from build123d import *

# Parameters (mm, degrees)
SKETCH_1_R          = 23
SKETCH_1_R_2        = 18
EXTRUDE_1_DEPTH     = 28
EXTRUDE_3_DEPTH     = 60
SKETCH_2_5_R        = 54
SKETCH_2_5_R_2      = 34
EXTRUDE_4_DEPTH     = 80
CUT_EXTRUDE_1_DEPTH = 30
SKETCH_6_W          = 108
SKETCH_6_H          = 28
EXTRUDE_5_DEPTH     = 60
EXTRUDE_6_DEPTH     = 15


with BuildPart() as part:
    # Sketch 1 → Extrude 1 (new body)
    with BuildSketch(Plane(origin=(0, 0, 0), x_dir=(1, 0, 0), z_dir=(0, 1, 0))):
        with BuildLine():
            Line((0, 40), (180, 40))
            ThreePointArc((180, 40), (220, 0), (180, -40))
            Line((180, -40), (0, -40))
            ThreePointArc((0, -40), (-40, 0), (0, 40))
        make_face()
        with Locations(Location((180, 0, 0), (0, 0, 270))):
            Circle(SKETCH_1_R, mode=Mode.SUBTRACT)
        with Locations(Location((0, 0, 0), (0, 0, 270))):
            Circle(SKETCH_1_R_2, mode=Mode.SUBTRACT)
    extrude(amount=EXTRUDE_1_DEPTH)



with BuildPart() as body_2:
    # Sketch 2 → Extrude 3 (new body)
    with BuildSketch(Plane(origin=(0, 28, 0), x_dir=(1, 0, 0), z_dir=(0, 1, 0))):
        with BuildLine():
            Line((90, 40), (144, 40))
            Line((144, 40), (144, 126))
            ThreePointArc((144, 126), (90, 72), (36, 126))
            Line((36, 126), (36, 40))
            Line((36, 40), (90, 40))
        make_face()
    extrude(amount=EXTRUDE_3_DEPTH)

    # Sketch 2_5 → Extrude 4 (add)
    with BuildSketch(Plane(origin=(0, 28, 0), x_dir=(1, 0, 0), z_dir=(0, 1, 0))):
        with Locations(Location((90, 126, 0), (0, 0, 180))):
            Circle(SKETCH_2_5_R)
        with Locations(Location((90, 126, 0), (0, 0, 270))):
            Circle(SKETCH_2_5_R_2, mode=Mode.SUBTRACT)
    extrude(amount=EXTRUDE_4_DEPTH)

    # Sketch 4 → Cut-Extrude 1 (cut)
    with BuildSketch(Plane.XZ.offset(-28)):
        with BuildLine():
            Line((36, -40), (36, -126))
            ThreePointArc((36, -126), (90, -180), (144, -126))
            Line((144, -126), (144, -40))
            Line((144, -40), (36, -40))
        make_face()
    extrude(amount=-CUT_EXTRUDE_1_DEPTH, mode=Mode.SUBTRACT)


with BuildPart() as part_1:
    add(part.part)

    add(body_2.part)  # Extrude 5 merges body 2
    # Sketch 6 → Extrude 5 (add)
    with BuildSketch(Plane(origin=(0, 28, 0), x_dir=(1, 0, 0), z_dir=(0, 1, 0))):
        with Locations((90, 26)):
            Rectangle(SKETCH_6_W, SKETCH_6_H)
    extrude(amount=EXTRUDE_5_DEPTH)

    # Sketch 7 → Extrude 6 (add, symmetric)
    with BuildSketch(Plane.ZY.offset(-90)):
        Polygon((40, 28), (-12, 28), (-12, 88), align=None)
    extrude(amount=EXTRUDE_6_DEPTH, both=True)


solid = part_1.part
Input: part model. Units: mm. Frame: model coordinates. A direction names the side the tool comes from. Coordinates: 2 decimals unless noted, no trailing zeros. Loops run counter-clockwise (first coordinate to the right, second up) from the corner with the lowest first, then second, coordinate; pieces in that order, holes last.
(1) Set-up query: faces 1 (the face through (101, 58, -93)), 2 (the face through (105, 45, 3)), 3 (the face through (144, 71, -56)), 4 (the face through (55, 58, -12)). Return all of +Z, -Z, +X, -X, +Y, -Y with unobstructed straight access to the full face (end or side cutting, diameter ignored); none if empty.
(2) First-contact query: pin 1 Ø10 at (y, z) = (75.5, -77.5) entering from +X; pin 2 Ø1.5 at (x, z) = (1, -41.5) entering from +Y; pin 3 Ø8 at (x, z) = (67.5, -149.5) entering from +Y; pin 4 Ø5 at (x, y) = (100.5, 89) entering from -Z. Flat tips, straight axial feed; report the tip coordinate or a pass-through.
(3) Pull-direction query (Z, two-part tool) for faces 5 (the face through (219.99, 13.8, -0.88)), 6 (the face through (55, 108, -125)), 7 (the face through (157.547, 13.804, -4.986)); classes: released by +Z, released by -Z, zero draft, split by the parting line, or undercut.
(4) Section D-D on y = 45. Return the cut outline in (x, z).
(5) Section C-C on z = 0. Return the cut outline in (x, y), then the cut area to 3 significant figures.
(6) Material intervals for probe 1 along X at (y, z) = (21.75, 0); probe 2 along Z at (x, y) = (90, 96); probe 3 along X at (y, z) = (81, -126), sorted ascending.
(7) Section A-A on x = 90. Return the cut outline in (y, z), then the cut area to 3 significant figures.
(8) Section B-B on z = -152.5. Return the cut outline in (x, y), then the cut area to 3 significant figures.
Data:
1. face 1: -Z, +X, -X, -Y
1. face 2: +Z, +X, +Y
1. face 3: +Z, -Z, +X, +Y
1. face 4: +Z, -X, +Y
2. pin 1: stops at x = 144
2. pin 2: passes through
2. pin 3: stops at y = 108
2. pin 4: stops at z = -179.4
3. face 5: split by the parting line
3. face 6: zero draft
3. face 7: undercut
4. outline: (36, -40) - (144, -40) - (144, -12) - (105, -12) - (105, 25.27) - (75, 25.27) - (75, -12) - (36, -12) - close
5. outline: (-40, 0) - (-18, 0) - (-18, 28) - (-40, 28) - close; (18, 0) - (157, 0) - (157, 28) - (105, 28) - (105, 74.15) - (75, 74.15) - (75, 28) - (18, 28) - close; (203, 0) - (220, 0) - (220, 28) - (203, 28) - close
5. area: 6,370 mm2
6. probe 1: x = -40 to -18, 18 to 157, 203 to 220
6. probe 2: z = -180 to -160, -92 to -72
6. probe 3: x = 36 to 56, 124 to 144
7. outline: (0, -40) - (58, -40) - (58, -92) - (108, -92) - (108, -72) - (88, -72) - (88, -12) - (28, 40) - (0, 40) - close; (58, -180) - (108, -180) - (108, -160) - (58, -160) - close
7. area: 8,440 mm2
8. outline: (42.95, 58) - (68.7, 58) - (68.7, 108) - (42.95, 108) - close; (111.3, 58) - (137.05, 58) - (137.05, 108) - (111.3, 108) - close
8. area: 2,570 mm2
